Geometry: final body of the model. Coordinates: model frame, mm. A direction names the side the tool comes from. Round coordinates to 2 decimals unless told otherwise and drop trailing zeros. Loops run counter-clockwise (first coordinate to the right, second up) from the corner with the lowest first, then second, coordinate; pieces in that order, holes last. Notation, with made-up numbers: (81, 24.5) -> (114, 24.5) arc R33 ccw to (114, 52.5) -> close; hole circle Ø4 at (70, 77). An arc over 180 degrees is marked (long way). Answer in a Markdown table with one row per item.
```python
from build123d import *

# Parameters (mm, degrees)
SKETCH1_R           = 2.5
BOSS_EXTRUDE2_DEPTH = 25.5
SKETCH2_R           = 3.5
BOSS_EXTRUDE3_DEPTH = 3
CUT_EXTRUDE2_DEPTH  = 2
CHAMFER2_SIZE       = 0.5
FILLET5_R           = 0.5


with BuildPart() as part:
    # Sketch1 → Boss-Extrude2 (new body)
    with BuildSketch(Plane.XY):
        Circle(SKETCH1_R)
    extrude(amount=BOSS_EXTRUDE2_DEPTH)

    # Sketch2 → Boss-Extrude3 (add)
    with BuildSketch(Plane(origin=(0, 0, 0), x_dir=(-1, 0, 0), z_dir=(0, 0, -1))):
        Circle(SKETCH2_R)
    extrude(amount=BOSS_EXTRUDE3_DEPTH)

    # Sketch4 → Cut-Extrude2 (cut)
    with BuildSketch(Plane(origin=(0, 0, -3), x_dir=(-1, 0, 0), z_dir=(0, 0, -1))):
        Polygon((2.180058464, 0), (0, 0), (0, -2.517314682), (2.180058464, -1.258657341), align=None)
        Polygon((2.180058464, 1.258657341), (0, 2.517314682), (0, 0), (2.180058464, 0), align=None)
        Polygon((0, 0), (0, 2.517314682), (-2.180058464, 1.258657341), (-2.180058464, 0), align=None)
        Polygon((0, -2.517314682), (0, 0), (-2.180058464, 0), (-2.180058464, -1.258657341), align=None)
    extrude(amount=-CUT_EXTRUDE2_DEPTH, mode=Mode.SUBTRACT)

    # Chamfer2
    chamfer2_edges = [part.edges().sort_by_distance(p)[0] for p in [
        (3.5, 0, -3),
    ]]
    chamfer(chamfer2_edges, length=CHAMFER2_SIZE)

    # Fillet5
    fillet5_edges = [part.edges().sort_by_distance(p)[0] for p in [
        (3.5, 0, 0),
    ]]
    fillet(fillet5_edges, radius=FILLET5_R)


solid = part.part
```
Item 1: Section query A-A, the plane y = 0. Output: boundary loops of the cut face in (x, z), and give its area (3 significant figures).
Ans:
| item | result |
|---|---|
| outline | (-3.5, -2.5) -> (-3, -3) -> (-2.18, -3) -> (-2.18, -1) -> (2.18, -1) -> (2.18, -3) -> (3, -3) -> (3.5, -2.5) -> (3.5, -0.5) arc R0.5 ccw to (3, 0) -> (2.5, 0) -> (2.5, 25.5) -> (-2.5, 25.5) -> (-2.5, 0) -> (-3, 0) arc R0.5 ccw to (-3.5, -0.5) -> close |
| area | 139 mm2 |
Item 2: First-contact query: P1, Ø1.5, axis at x = 0, z = 12, coming from the +Y side; P2, Ø2, axis at y = -2.5, z = 11, coming from the -X side; P3, Ø2, axis at x = 2, y = 0.5, coming from the -Z side; P4, Ø2, axis at x = -0.5, y = -1, coming from the -Z side. Flat tips, straight axial feed; report the tip coordinate or a pass-through.
Ans:
| item | result |
|---|---|
| P1 | y = 2.5 |
| P2 | x = -2 |
| P3 | z = -3 |
| P4 | z = -1 |
Item 3: Section query B-B, the plane z = 13.25. Output: boundary loops of the cut face in (x, y).
Ans:
| item | result |
|---|---|
| outline | circle Ø5 at (0, 0) |
Item 4: Mould query, pull axis Y, two halves, no side actions, for faces 1 (the flat face through (0, 0, 25.5)), 2 (the cylindrical face through (-3.233, -1.341, -1.486)), 3 (the flat face through (-1.105, 1.879, -2.014)). Classes: released by +Y, released by -Y, zero draft, split by the parting line, or undercut.
Ans:
| item | result |
|---|---|
| face 1 | zero draft |
| face 2 | split by the parting line |
| face 3 | undercut |
Item 5: Set-up query: faces 4 (the flat face through (2, 2, 0)), 5 (the flat face through (2.18, 0, -2)). Return all of +Z, -Z, +X, -X, +Y, -Y with unobstructed straight access to the full face (end or side cutting, diameter ignored); none if empty.
Ans:
| item | result |
|---|---|
| face 4 | +Z |
| face 5 | -Z |
Item 6: Ray query, L1, parallel to Z at x = 0, y = -1.75; L2, parallel to Z at x = 2.5, y = 0.5; L3, parallel to Y at x = 0, z = 9. Return the intervals inside material, ascending.
Ans:
| item | result |
|---|---|
| L1 | -1 to 25.5 |
| L2 | -3 to 0 |
| L3 | -2.5 to 2.5 |
